```python
from build123d import *

# Parameters (mm, degrees)
SKETCH1_W             = 38
SKETCH1_H             = 52
EXTRUDE1_DEPTH        = 22
SKETCH2_R             = 2.925
CUT_EXTRUDE1_DEPTH    = 12.7
SKETCH5_W             = 12
SKETCH5_H             = 22
CUT_EXTRUDE4_DEPTH    = 4
F_8_CLEARANCE_HOLE1_D = 4.3053
CUT_EXTRUDE5_REACH    = 61.573
SKETCH8_R             = 0.508
SKETCH9_W             = 0.25
SKETCH9_H             = 22
CUT_EXTRUDE6_DEPTH    = 0.1


with BuildPart() as part:
    # Sketch1 → Extrude1 (new body)
    with BuildSketch(Plane.XY):
        with Locations((0, 26)):
            Rectangle(SKETCH1_W, SKETCH1_H)
    extrude(amount=EXTRUDE1_DEPTH)

    # Sketch2 → Cut-Extrude1 (cut)
    with BuildSketch(Plane(origin=(0, 52, 0), x_dir=(-1, 0, 0), z_dir=(0, 1, 0))):
        with Locations(Location((12.5, 5, 0), (0, 0, 90))):
            Circle(SKETCH2_R)
        with Locations(Location((12.5, 17, 0), (0, 0, 270))):
            Circle(SKETCH2_R)
        with Locations(Location((-12.5, 17, 0), (0, 0, 90))):
            Circle(SKETCH2_R)
        with Locations(Location((-12.5, 5, 0), (0, 0, 270))):
            Circle(SKETCH2_R)
    extrude(amount=-CUT_EXTRUDE1_DEPTH, mode=Mode.SUBTRACT)

    # Sketch5 → Cut-Extrude4 (cut)
    with BuildSketch(Plane(origin=(0, 52, 0), x_dir=(-1, 0, 0), z_dir=(0, 1, 0))):
        with Locations((0, 11)):
            Rectangle(SKETCH5_W, SKETCH5_H)
    extrude(amount=-CUT_EXTRUDE4_DEPTH, mode=Mode.SUBTRACT)

    # #8 Clearance Hole1 (through all)
    with Locations(Plane(origin=(0, 48, 0), x_dir=(-1, 0, 0), z_dir=(0, 1, 0))):
        with Locations((0, 17), (0, 5)):
            Hole(F_8_CLEARANCE_HOLE1_D / 2)

    # Sketch8 → Cut-Extrude5 (cut, up to next)
    with BuildSketch(Plane.XY.offset(22), mode=Mode.PRIVATE) as cut_extrude5_sk1:
        with Locations((-12.5, 42.475)):
            Circle(SKETCH8_R)
    cut_extrude5_tool1 = extrude(cut_extrude5_sk1.sketch, amount=-CUT_EXTRUDE5_REACH, mode=Mode.PRIVATE) & part.part
    # Sketch8 → Cut-Extrude5 (cut, up to next)
    with BuildSketch(Plane.XY.offset(22), mode=Mode.PRIVATE) as cut_extrude5_sk2:
        with Locations((12.5, 42.475)):
            Circle(SKETCH8_R)
    cut_extrude5_tool2 = extrude(cut_extrude5_sk2.sketch, amount=-CUT_EXTRUDE5_REACH, mode=Mode.PRIVATE) & part.part
    cut_extrude5_1 = cut_extrude5_tool1.solids().sort_by_distance((-12.5, 42.475, 22))[0]
    add(cut_extrude5_1, mode=Mode.SUBTRACT)
    cut_extrude5_2 = cut_extrude5_tool2.solids().sort_by_distance((12.5, 42.475, 22))[0]
    add(cut_extrude5_2, mode=Mode.SUBTRACT)
    cut_extrude5 = cut_extrude5_1 + cut_extrude5_2  # Cut-Extrude5 as one shape, for the pattern or mirror that repeats it

    # Mirror1: Cut-Extrude5 mirrored; each copy of Cut-Extrude5 runs up to whatever stops it at its own place
    mirror1_before = part.part  # the part as the pattern finds it: every copy runs up to it
    mirror1_cut_extrude5_long1 = extrude(cut_extrude5_sk1.sketch, amount=-CUT_EXTRUDE5_REACH, mode=Mode.PRIVATE)
    mirror1_cut_extrude5_long2 = extrude(cut_extrude5_sk2.sketch, amount=-CUT_EXTRUDE5_REACH, mode=Mode.PRIVATE)
    mirror1_cut_extrude5_tool = mirror1_cut_extrude5_long1.mirror(Plane.XY) & mirror1_before
    add(mirror1_cut_extrude5_tool.solids().sort_by_distance((-12.5, 42.475, -22))[0], mode=Mode.SUBTRACT)
    mirror1_cut_extrude5_tool = mirror1_cut_extrude5_long2.mirror(Plane.XY) & mirror1_before
    add(mirror1_cut_extrude5_tool.solids().sort_by_distance((12.5, 42.475, -22))[0], mode=Mode.SUBTRACT)

    # Sketch9 → Cut-Extrude6 (cut)
    with BuildSketch(Plane(origin=(0, 48, 0), x_dir=(-1, 0, 0), z_dir=(0, 1, 0))):
        with Locations((0, 11)):
            Rectangle(SKETCH9_W, SKETCH9_H)
    extrude(amount=-CUT_EXTRUDE6_DEPTH, mode=Mode.SUBTRACT)


solid = part.part
```
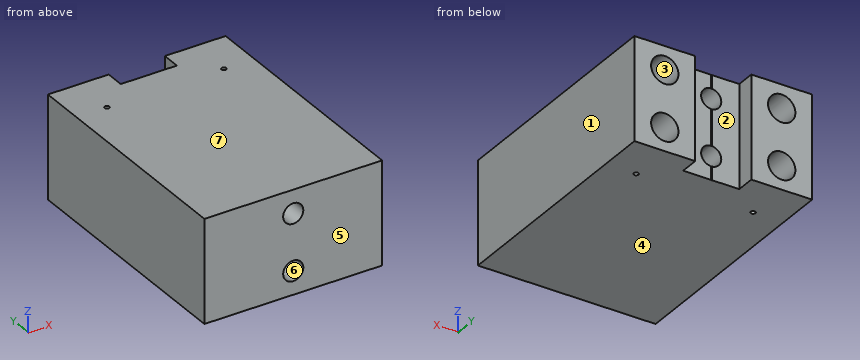
CAD build for the part. Positions are in the model's coordinates, mm. Face numbers are marked on the shaded views. A direction names the side the tool comes from. Round coordinates to 2 decimals unless told otherwise and drop trailing zeros. Write each loop counter-clockwise with the first axis right and the second up, starting at its lowest first coordinate (ties: lowest second). Pieces come first, ordered by that corner, then holes.
Item 1: Tool access for the marked faces 1, 2 and 3: list every direction of +Z, -Z, +X, -X, +Y, -Y with a clear straight run to the whole face (end or side of a thin tool).
Filled in:
face 1: +Z, -Z, +X, +Y, -Y
face 2: +Z, -Z, +Y
face 3: +Y
Item 2: Band-saw the part on C-C on z = 10. Write the cut outline in (x, y) (3 decimals).
Filled in:
outline: (-19, 0) - (19, 0) - (19, 52) - (6, 52) - (6, 48) - (0.125, 48) - (0.125, 47.9) - (-0.125, 47.9) - (-0.125, 48) - (-6, 48) - (-6, 52) - (-19, 52) - close
Item 3: Band-saw the part on A-A on z = 5. Write the cut outline in (x, y) (3 decimals), then the cut area to 3 significant figures.
Filled in:
outline: (-19, 0) - (-2.153, 0) - (-2.153, 48) - (-6, 48) - (-6, 52) - (-9.575, 52) - (-9.575, 39.3) - (-15.425, 39.3) - (-15.425, 52) - (-19, 52) - close; (2.153, 0) - (19, 0) - (19, 52) - (15.425, 52) - (15.425, 39.3) - (9.575, 39.3) - (9.575, 52) - (6, 52) - (6, 48) - (2.153, 48) - close
area: 1,570 mm2
Item 4: Band-saw the part on D-D on y = 18. Write the cut outline in (x, z).
Filled in:
outline: (-19, 0) - (19, 0) - (19, 22) - (-19, 22) - close; hole circle Ø4.31 at (0, 5); hole circle Ø4.31 at (0, 17)
Item 5: Band-saw the part on B-B on y = 47. Write the cut outline in (x, z) (3 decimals), then the cut area to 3 significant figures.
Filled in:
outline: (-19, 0) - (19, 0) - (19, 22) - (-19, 22) - close; hole circle Ø5.85 at (-12.5, 5); hole circle Ø5.85 at (-12.5, 17); hole circle Ø4.305 at (0, 5); hole circle Ø4.305 at (0, 17); hole circle Ø5.85 at (12.5, 5); hole circle Ø5.85 at (12.5, 17)
area: 699 mm2
Item 6: Drop flat-ended pins along their axis: pin 1 Ø1.8 at (x, z) = (-13, 15.5) entering from +Y; pin 2 Ø5 at (x, z) = (0, 17) entering from +Y; pin 3 Ø0.8 at (x, y) = (12.5, 42.475) entering from -Z. Give the stop position or say it passes through.
Filled in:
pin 1: stops at y = 39.3
pin 2: stops at y = 48
pin 3: stops at z = 7.9
Item 7: Drill centre lines: L1, parallel to Z at x = 0, y = 13; L2, parallel to X at y = 42.5, z = 17 (3 decimals); L3, parallel to Z at x = -11, y = 41. Where is each one in solid material? Low to high.
Filled in:
L1: z = 0 to 2.85, 7.15 to 14.85, 19.15 to 22
L2: x = -19 to -15.425, -9.575 to -2.153, 2.153 to 9.575, 15.425 to 19
L3: z = 0 to 2.49, 7.51 to 14.49, 19.51 to 22
Item 8: Mould opens along Z. For the marked faces 4, 5, 6 and 7 say: released by +Z, released by -Z, zero draft, split by the parting line, or undercut.
Filled in:
face 4: released by -Z
face 5: zero draft
face 6: undercut
face 7: released by +Z
